Source: three-view drawing plus pictorial views. Frame: mm from the lowest corner of the part. Coordinates: 2 decimals unless noted, no trailing zeros. Loops run counter-clockwise (first coordinate to the right, second up) from the corner with the lowest first, then second, coordinate; pieces in that order, holes last. Notation, with made-up numbers: (49.25, 81) - (60.25, 81) arc R21 cw to (60.25, 103) - close; hole circle Ø6 at (77, 55). An arc over 180 degrees is marked (long way). Answer as CSV lines item,"result". Start each with the question number.
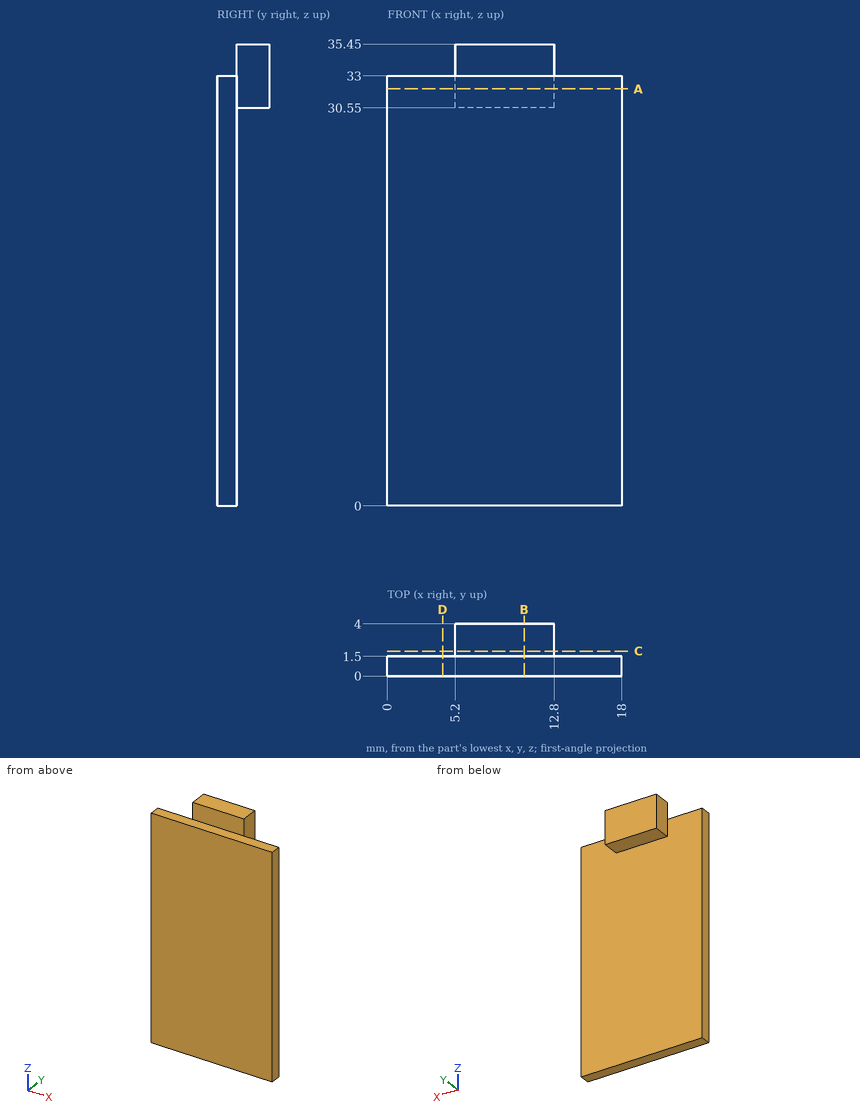
Item 1: Section query C-C, the plane y = 1.9. Output: boundary loops of the cut face in (x, z).
Item 2: Section query B-B, the plane x = 10.5. Output: boundary loops of the cut face in (y, z).
Item 3: Contact query for flat-ended pins moving along their axis: P1, Ø2, axis at y = 3, z = 32, coming from the -X side; P2, Ø4, axis at x = 13, z = 24, coming from the -Y side; P3, Ø2.5, axis at x = 8, z = 35, coming from the -Y side; P4, Ø0.8, axis at y = 2.5, z = 33.5, coming from the +X side. Output: stop coordinate, or through.
Item 4: Section query A-A, the plane z = 32. Output: boundary loops of the cut face in (x, y).
Item 5: Material intervals for probe 1 along Y at (x, z) = (6.5, 26.5); probe 2 along Z at (x, y) = (4.75, 0.95); probe 3 along X at (y, z) = (2.8, 31), sorted ascending.
Item 6: Section query D-D, the plane x = 4.25. Output: boundary loops of the cut face in (y, z), and give its area (3 significant figures).
Response values:
1,outline,"(5.2, 30.55) - (12.8, 30.55) - (12.8, 35.45) - (5.2, 35.45) - close"
2,outline,"(0, 0) - (1.5, 0) - (1.5, 30.55) - (4, 30.55) - (4, 35.45) - (1.5, 35.45) - (1.5, 33) - (0, 33) - close"
3,P1,"stops at x = 5.2"
3,P2,"stops at y = 0"
3,P3,"stops at y = 1.5"
3,P4,"stops at x = 12.8"
4,outline,"(0, 0) - (18, 0) - (18, 1.5) - (12.8, 1.5) - (12.8, 4) - (5.2, 4) - (5.2, 1.5) - (0, 1.5) - close"
5,probe 1,"y = 0 to 1.5"
5,probe 2,"z = 0 to 33"
5,probe 3,"x = 5.2 to 12.8"
6,outline,"(0, 0) - (1.5, 0) - (1.5, 33) - (0, 33) - close"
6,area,"49.5 mm²"
